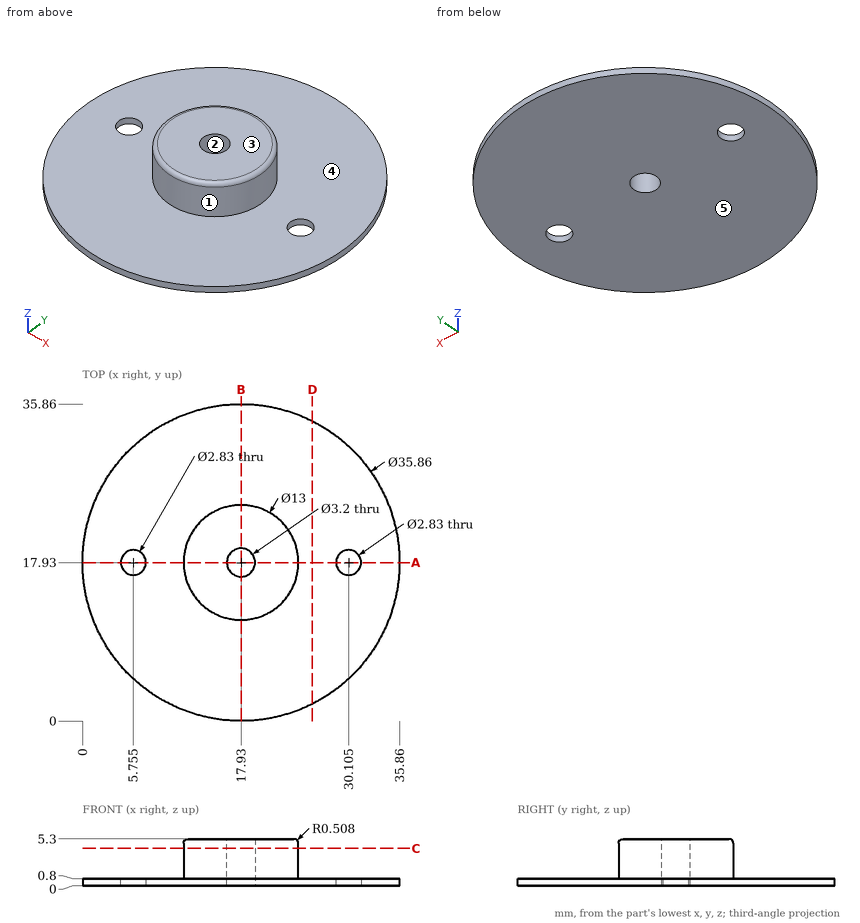
Drawing for the job (mm, zero at the part's lowest x, y, z). A direction names the side the tool comes from. Round coordinates to 2 decimals unless told otherwise and drop trailing zeros. Write each loop counter-clockwise with the first axis right and the second up, starting at its lowest first coordinate (ties: lowest second). Pieces come first, ordered by that corner, then holes. Notation, with made-up numbers: (-31, 49.5) - (-4, 49.5) arc R12 ccw to (-4, 53.5) - close; hole circle Ø10 at (56, 43). An arc over 180 degrees is marked (long way). Return JSON: item names as keys, results as strings. Group by question number.
Item 1: 3-axis set-ups, long thin cutter, end or side, ignore diameter. For the marked faces 4 and 5: which of +Z, -Z, +X, -X, +Y, -Y reach the whole face in a straight line?
Item 2: Flat gauge pins, fed straight in: pin 1 Ø6 at (x, y) = (7.5, 4.5) entering from +Z; pin 2 Ø1.7 at (x, y) = (5.755, 17.93) entering from +Z. Where does each tip first touch, or does it go through?
Item 3: Band-saw the part on B-B on x = 17.93. List the corners of the cut face in (y, z).
Item 4: Probe probe 1 along Z at (x, y) = (21, 26.5); probe 2 along Y at (x, z) = (19, 3.1); probe 3 along X at (y, z) = (13, 2.85). List the from-to ranges inside material, lowest first.
Item 5: Band-saw the part on A-A on y = 17.93. List the corners of the cut face in (x, z), plus the area to 3 significant figures.
Item 6: Band-saw the part on D-D on x = 26. List the corners of the cut face in (y, z), plus the area to 3 significant figures.
Item 7: Mould opens along Y. For the marked faces 1, 2 and 3 say: +Y half, -Y half, draft (parallel to the pull), parting line (faces both ways), or undercut.
Item 8: Band-saw the part on C-C on z = 4.25. List the corners of the cut face in (x, y).
Resolved:
{
 "1": {"face 4": "+Z", "face 5": "-Z, +X, -X, +Y, -Y"},
 "2": {"pin 1": "stops at z = 0.8", "pin 2": "passes through"},
 "3": {"outline": "(0, 0) - (16.33, 0) - (16.33, 5.3) - (11.94, 5.3) arc R0.51 ccw to (11.43, 4.79) - (11.43, 0.8) - (0, 0.8) - close; (19.53, 0) - (35.86, 0) - (35.86, 0.8) - (24.43, 0.8) - (24.43, 4.79) arc R0.51 ccw to (23.92, 5.3) - (19.53, 5.3) - close"},
 "4": {"probe 1": "z = 0 to 0.8", "probe 2": "y = 11.52 to 16.74, 19.12 to 24.34", "probe 3": "x = 13.69 to 22.17"},
 "5": {"outline": "(0, 0) - (4.34, 0) - (4.34, 0.8) - (0, 0.8) - close; (7.17, 0) - (16.33, 0) - (16.33, 5.3) - (11.94, 5.3) arc R0.51 ccw to (11.43, 4.79) - (11.43, 0.8) - (7.17, 0.8) - close; (19.53, 0) - (28.69, 0) - (28.69, 0.8) - (24.43, 0.8) - (24.43, 4.79) arc R0.51 ccw to (23.92, 5.3) - (19.53, 5.3) - close; (31.52, 0) - (35.86, 0) - (35.86, 0.8) - (31.52, 0.8) - close", "area": "65.6 mm²"},
 "6": {"outline": "(1.92, 0) - (33.94, 0) - (33.94, 0.8) - (1.92, 0.8) - close", "area": "25.6 mm²"},
 "7": {"face 1": "parting line", "face 2": "undercut", "face 3": "draft"},
 "8": {"outline": "circle Ø13 at (17.93, 17.93); hole circle Ø3.2 at (17.93, 17.93)"}
}
